Autodesk Inventor part; units mm, degrees
ref_plane "YZ Plane" through (0, 0, 0) normal (1, 0, 0) x (0, 1, 0)
ref_plane "XZ Plane" through (0, 0, 0) normal (0, 1, 0) x (-1, 0, 0)
ref_plane "XY Plane" through (0, 0, 0) normal (0, 0, 1) x (1, 0, 0)
sketch "Esquisse1" plane through (0, 0, 0) normal (0, 1, 0) x (-1, 0, 0)
  line L0 (110.1985, 107.2202) -> (-139.8015, 107.2202)
  line L1 (-139.8015, 107.2202) -> (-139.8015, -192.7798)
  line L2 (-139.8015, -192.7798) -> (110.1985, -192.7798)
  line L3 (110.1985, -192.7798) -> (110.1985, 107.2202)
  point P0 (0, 0)
  dimension "d0" = 300
  dimension "d1" = 250
extrude "Extrusion1" add sketch "Esquisse1" along normal blind 5
sketch "Esquisse2" plane through (0, 0, 0) normal (0, -1, 0) x (1, 0, 0)
  circle A0 centre (-94.1985, -42.7798) radius 1.5
  circle A1 centre (123.8015, -42.7798) radius 1.5
  circle A2 centre (123.8015, 67.2202) radius 1.5
  circle A3 centre (123.8015, -152.7798) radius 1.5
  line L0 (-110.1985, -192.7798) -> (-110.1985, 107.2202)
  line L1 (139.8015, -192.7798) -> (-110.1985, -192.7798)
  line L2 (139.8015, 107.2202) -> (139.8015, -192.7798)
  line L3 (-110.1985, 107.2202) -> (139.8015, 107.2202)
  point P0 (0, 0)
  dimension "d4" = 16
  dimension "d5" = 150
  dimension "d6" = 16
  dimension "d7" = 16
  dimension "d8" = 16
  dimension "d9" = 40
  dimension "d10" = 150
  dimension "d11" = 40
extrude "Extrusion2" cut sketch "Esquisse2" against normal through all contours A0 | A1 | A2 | A3
sketch "Esquisse6" plane through (0, 0, 0) normal (0, -1, 0) x (1, 0, 0)
  circle A0 centre (-90.1985, 77.2202) radius 7.5
  line L0 (-110.1985, 107.2202) -> (139.8015, 107.2202)
  line L1 (-110.1985, -192.7798) -> (-110.1985, 107.2202)
  point P0 (0, 0)
  dimension "d32" = 15
  dimension "d33" = 30
  dimension "d34" = 20
extrude "Extrusion6" cut sketch "Esquisse6" against normal up to next
sketch "Esquisse7" plane through (0, 0, 0) normal (0, -1, 0) x (1, 0, 0)
  circle A0 centre (-17.1985, -10.7798) radius 2
  circle A1 centre (-17.1985, -74.7798) radius 2
  circle A2 centre (46.8015, -74.7798) radius 2
  circle A3 centre (46.8015, -10.7798) radius 2
  point P0 (0, 0)
extrude "Extrusion7" cut sketch "Esquisse7" against normal up to next
properties part number "toit"
Input: part model. Units: mm. Frame: model coordinates. Round coordinates to 2 decimals unless told otherwise and drop trailing zeros. Loops run counter-clockwise (first coordinate to the right, second up) from the corner with the lowest first, then second, coordinate; pieces in that order, holes last. Notation, with made-up numbers: (-28.75, 63.25) -> (29.25, 63.25) arc R19 cw to (29.25, 83.25) -> close; hole circle Ø8 at (-16.5, 0.25). An arc over 180 degrees is marked (long way). Use one line per item in the form item = value. Start each with the question number.
Item 1: Section query B-B on x = -86.5. Return the cut outline in (y, z).
Item 2: Section query A-A on z = 73.5. Return the cut outline in (x, y), then the cut area to 3 significant figures.
Item 3: Material intervals for L1, parallel to Z at x = -16, y = 2.05; L2, parallel to X at y = 1.8, z = -44, sorted ascending. Write a range as from..to.
Item 4: Contact query for flat-ended pins moving along their axis: pin 1 Ø5 at (x, z) = (-94.2, -42.78) entering from +Y; pin 2 Ø13.5 at (x, z) = (-90.2, 77.22) entering from +Y. Output: stop coordinate, or through.
Item 5: Mould query, pull axis X, two halves, no side actions, for faces 1 (the face through (-83.27, 2.46, 74.35)), 2 (the face through (17, 5, -41)). Classes: pulls with the +X half, pulls with the -X half, needs draft (parallel to the pull), parting line crosses it, or undercut.
Ans:
q1.outline = (0, -192.78) -> (5, -192.78) -> (5, 70.7) -> (0, 70.7) -> close; (0, 83.74) -> (5, 83.74) -> (5, 107.22) -> (0, 107.22) -> close
q2.outline = (-110.2, 0) -> (-96.71, 0) -> (-96.71, 5) -> (-110.2, 5) -> close; (-83.69, 0) -> (139.8, 0) -> (139.8, 5) -> (-83.69, 5) -> close
q2.area = 1,180 mm^2
q3.L1 = -192.78..-76.38, -73.18..-12.38, -9.18..107.22
q3.L2 = -110.2..-95.07, -93.33..122.93, 124.67..139.8
q4.pin_1 = 5
q4.pin_2 = through
q5.face_1 = undercut
q5.face_2 = needs draft
